The listing builds one solid part. Answer for the finished solid, in the listing's coordinates (mm). Give positions to 0.01 mm unless a question says otherwise; leave off trailing zeros. Order: outer loops, then holes, each group sorted by start corner. A loop starts at its lowest first (then second) coordinate and runs counter-clockwise, first axis right, second up. Notation, with made-up numbers: M 1.25,-11 L 29.25,-11 A17 cw 29.25,5 Z; hole C 68.25,-26.75 d8. An arc over 180 degrees is marked long. Answer as a JSON object with one key per item and string values. Group by question number.
```python
from build123d import *

# Parameters (mm, degrees)
MODEL_R             = 1.6
MODEL_R_2           = 3
MODEL_R_3           = 15
BOSS_EXTRUDE1_DEPTH = 1.5


with BuildPart() as part:
    # Model → Boss-Extrude1 (new, symmetric)
    with BuildSketch(Plane.XY):
        with BuildLine():
            Line((-87, -128), (87, -128))
            ThreePointArc((87, -128), (90.535533906, -126.535533906), (92, -123))
            Line((92, -123), (92, 123))
            ThreePointArc((92, 123), (90.535533906, 126.535533906), (87, 128))
            Line((87, 128), (-87, 128))
            ThreePointArc((-87, 128), (-90.535533906, 126.535533906), (-92, 123))
            Line((-92, 123), (-92, -123))
            ThreePointArc((-92, -123), (-90.535533906, -126.535533906), (-87, -128))
        make_face()
        with Locations((-75, 62)):
            Circle(MODEL_R, mode=Mode.SUBTRACT)
        with Locations((-32, 62)):
            Circle(MODEL_R, mode=Mode.SUBTRACT)
        with Locations((-75, -62)):
            Circle(MODEL_R, mode=Mode.SUBTRACT)
        with Locations((-32, -62)):
            Circle(MODEL_R, mode=Mode.SUBTRACT)
        with Locations((32, 62)):
            Circle(MODEL_R, mode=Mode.SUBTRACT)
        with Locations((75, 62)):
            Circle(MODEL_R, mode=Mode.SUBTRACT)
        with Locations((32, -62)):
            Circle(MODEL_R, mode=Mode.SUBTRACT)
        with Locations((75, -62)):
            Circle(MODEL_R, mode=Mode.SUBTRACT)
        with Locations((-39, 115)):
            Circle(MODEL_R, mode=Mode.SUBTRACT)
        with Locations((-39, 73)):
            Circle(MODEL_R, mode=Mode.SUBTRACT)
        with Locations((39, 115)):
            Circle(MODEL_R, mode=Mode.SUBTRACT)
        with Locations((39, 73)):
            Circle(MODEL_R, mode=Mode.SUBTRACT)
        with Locations((-39, -115)):
            Circle(MODEL_R, mode=Mode.SUBTRACT)
        with Locations((-39, -73)):
            Circle(MODEL_R, mode=Mode.SUBTRACT)
        with Locations((39, -115)):
            Circle(MODEL_R, mode=Mode.SUBTRACT)
        with Locations((39, -73)):
            Circle(MODEL_R, mode=Mode.SUBTRACT)
        Circle(MODEL_R_2, mode=Mode.SUBTRACT)
        with Locations((0, 15)):
            Circle(MODEL_R_2, mode=Mode.SUBTRACT)
        with Locations((0, -15)):
            Circle(MODEL_R_2, mode=Mode.SUBTRACT)
        with Locations((0, 42)):
            Circle(MODEL_R_3, mode=Mode.SUBTRACT)
        with Locations((0, -42)):
            Circle(MODEL_R_3, mode=Mode.SUBTRACT)
        with Locations((-75, 115)):
            Circle(MODEL_R, mode=Mode.SUBTRACT)
        with Locations((75, 115)):
            Circle(MODEL_R, mode=Mode.SUBTRACT)
        with Locations((-75, -115)):
            Circle(MODEL_R, mode=Mode.SUBTRACT)
        with Locations((75, -115)):
            Circle(MODEL_R, mode=Mode.SUBTRACT)
        with Locations((-69, 88.5)):
            Circle(MODEL_R_3, mode=Mode.SUBTRACT)
        with Locations((69, 88.5)):
            Circle(MODEL_R_3, mode=Mode.SUBTRACT)
        with Locations((-69, -88.5)):
            Circle(MODEL_R_3, mode=Mode.SUBTRACT)
        with Locations((69, -88.5)):
            Circle(MODEL_R_3, mode=Mode.SUBTRACT)
        with BuildLine():
            Line((-80.366563146, 62), (-82.4, 62))
            ThreePointArc((-82.4, 62), (-83.53137085, 61.53137085), (-84, 60.4))
            Line((-84, 60.4), (-84, -60.4))
            ThreePointArc((-84, -60.4), (-83.53137085, -61.53137085), (-82.4, -62))
            Line((-82.4, -62), (-80.366563146, -62))
            ThreePointArc((-80.366563146, -62), (-79.410380259, -61.682853961), (-78.83325939, -60.857142857))
            ThreePointArc((-78.83325939, -60.857142857), (-75, -58), (-71.16674061, -60.857142857))
            ThreePointArc((-71.16674061, -60.857142857), (-70.589619741, -61.682853961), (-69.633436854, -62))
            Line((-69.633436854, -62), (-37.366563146, -62))
            ThreePointArc((-37.366563146, -62), (-36.410380259, -61.682853961), (-35.83325939, -60.857142857))
            ThreePointArc((-35.83325939, -60.857142857), (-32, -58), (-28.16674061, -60.857142857))
            ThreePointArc((-28.16674061, -60.857142857), (-27.589619741, -61.682853961), (-26.633436854, -62))
            Line((-26.633436854, -62), (-24.6, -62))
            ThreePointArc((-24.6, -62), (-23.46862915, -61.53137085), (-23, -60.4))
            Line((-23, -60.4), (-23, 60.4))
            ThreePointArc((-23, 60.4), (-23.46862915, 61.53137085), (-24.6, 62))
            Line((-24.6, 62), (-26.633436854, 62))
            ThreePointArc((-26.633436854, 62), (-27.589619741, 61.682853961), (-28.16674061, 60.857142857))
            ThreePointArc((-28.16674061, 60.857142857), (-32, 58), (-35.83325939, 60.857142857))
            ThreePointArc((-35.83325939, 60.857142857), (-36.410380259, 61.682853961), (-37.366563146, 62))
            Line((-37.366563146, 62), (-69.633436854, 62))
            ThreePointArc((-69.633436854, 62), (-70.589619741, 61.682853961), (-71.16674061, 60.857142857))
            ThreePointArc((-71.16674061, 60.857142857), (-75, 58), (-78.83325939, 60.857142857))
            ThreePointArc((-78.83325939, 60.857142857), (-79.410380259, 61.682853961), (-80.366563146, 62))
        make_face(mode=Mode.SUBTRACT)
        with BuildLine():
            Line((26.633436854, 62), (24.6, 62))
            ThreePointArc((24.6, 62), (23.46862915, 61.53137085), (23, 60.4))
            Line((23, 60.4), (23, -60.4))
            ThreePointArc((23, -60.4), (23.46862915, -61.53137085), (24.6, -62))
            Line((24.6, -62), (26.633436854, -62))
            ThreePointArc((26.633436854, -62), (27.589619741, -61.682853961), (28.16674061, -60.857142857))
            ThreePointArc((28.16674061, -60.857142857), (32, -58), (35.83325939, -60.857142857))
            ThreePointArc((35.83325939, -60.857142857), (36.410380259, -61.682853961), (37.366563146, -62))
            Line((37.366563146, -62), (69.633436854, -62))
            ThreePointArc((69.633436854, -62), (70.589619741, -61.682853961), (71.16674061, -60.857142857))
            ThreePointArc((71.16674061, -60.857142857), (75, -58), (78.83325939, -60.857142857))
            ThreePointArc((78.83325939, -60.857142857), (79.410380259, -61.682853961), (80.366563146, -62))
            Line((80.366563146, -62), (82.4, -62))
            ThreePointArc((82.4, -62), (83.53137085, -61.53137085), (84, -60.4))
            Line((84, -60.4), (84, 60.4))
            ThreePointArc((84, 60.4), (83.53137085, 61.53137085), (82.4, 62))
            Line((82.4, 62), (80.366563146, 62))
            ThreePointArc((80.366563146, 62), (79.410380259, 61.682853961), (78.83325939, 60.857142857))
            ThreePointArc((78.83325939, 60.857142857), (75, 58), (71.16674061, 60.857142857))
            ThreePointArc((71.16674061, 60.857142857), (70.589619741, 61.682853961), (69.633436854, 62))
            Line((69.633436854, 62), (37.366563146, 62))
            ThreePointArc((37.366563146, 62), (36.410380259, 61.682853961), (35.83325939, 60.857142857))
            ThreePointArc((35.83325939, 60.857142857), (32, 58), (28.16674061, 60.857142857))
            ThreePointArc((28.16674061, 60.857142857), (27.589619741, 61.682853961), (26.633436854, 62))
        make_face(mode=Mode.SUBTRACT)
        with BuildLine():
            Line((34, 113.6), (34, 74.4))
            ThreePointArc((34, 74.4), (33.121320344, 72.278679656), (31, 71.4))
            Line((31, 71.4), (-31, 71.4))
            ThreePointArc((-31, 71.4), (-33.121320344, 72.278679656), (-34, 74.4))
            Line((-34, 74.4), (-34, 113.6))
            ThreePointArc((-34, 113.6), (-33.121320344, 115.721320344), (-31, 116.6))
            Line((-31, 116.6), (31, 116.6))
            ThreePointArc((31, 116.6), (33.121320344, 115.721320344), (34, 113.6))
        make_face(mode=Mode.SUBTRACT)
        with BuildLine():
            Line((34, -113.6), (34, -74.4))
            ThreePointArc((34, -74.4), (33.121320344, -72.278679656), (31, -71.4))
            Line((31, -71.4), (-31, -71.4))
            ThreePointArc((-31, -71.4), (-33.121320344, -72.278679656), (-34, -74.4))
            Line((-34, -74.4), (-34, -113.6))
            ThreePointArc((-34, -113.6), (-33.121320344, -115.721320344), (-31, -116.6))
            Line((-31, -116.6), (31, -116.6))
            ThreePointArc((31, -116.6), (33.121320344, -115.721320344), (34, -113.6))
        make_face(mode=Mode.SUBTRACT)
    extrude(amount=BOSS_EXTRUDE1_DEPTH, both=True)


solid = part.part
```
Item 1: Consider probe 1 along X at (y, z) = (-115, 0.6); probe 2 along Y at (x, z) = (-39, 0.25); probe 3 along Y at (x, z) = (-20, 0.4). Determine where each line is inside the solid, lowest interval first. Write a range as from..to.
Item 2: Section C-C (y = 100.5) is taken. Determine the outline of the cut face in (x, z).
Item 3: A flat-ended cylindrical pin translates along its axis: P1, Ø2.5, axis at x = 32, y = -62, coming from the +Z side. Find the tip coordinate at first contact, or state that the pin passes through.
Item 4: Section A-A (y = -15) is taken. Determine the outline of the cut face in (x, z), and give its area (3 significant figures).
Item 5: Section B-B (x = 46) is taken. Determine the outline of the cut face in (y, z).
Item 6: Determine the mould class of faces 1 (the cylindrical face through (-1.953, -27.128, -0.021)), 2 (the cylindrical face through (-91, -126, 0)), 3 (the flat face through (6, 1, -1.5)), 4 (the cylindrical face through (65.748, -103.143, -0.021)) for opening direction X: released by +X, released by -X, zero draft, split by the parting line, or undercut.
Item 7: Section D-D (z = -0.95) is taken. Count the separate pieces of the cut face and the enclosed holes in it, and give its area (3 significant figures).
Values found:
{
 "1": {"probe 1": "x = -92..-76.6, -73.4..-40.6, -37.4..-33.65, 33.65..37.4, 40.6..73.4, 76.6..92", "probe 2": "y = -128..-116.6, -113.4..-74.6, -71.4..-62, 62..71.4, 74.6..113.4, 116.6..128", "probe 3": "y = -128..-116.6, -71.4..71.4, 116.6..128"},
 "2": {"outline": "M -92,-1.5 L -78,-1.5 L -78,1.5 L -92,1.5 Z; M -60,-1.5 L -34,-1.5 L -34,1.5 L -60,1.5 Z; M 34,-1.5 L 60,-1.5 L 60,1.5 L 34,1.5 Z; M 78,-1.5 L 92,-1.5 L 92,1.5 L 78,1.5 Z"},
 "3": {"P1": "passes through"},
 "4": {"outline": "M -92,-1.5 L -84,-1.5 L -84,1.5 L -92,1.5 Z; M -23,-1.5 L -3,-1.5 L -3,1.5 L -23,1.5 Z; M 3,-1.5 L 23,-1.5 L 23,1.5 L 3,1.5 Z; M 84,-1.5 L 92,-1.5 L 92,1.5 L 84,1.5 Z", "area": "168 mm^2"},
 "5": {"outline": "M -128,-1.5 L -62,-1.5 L -62,1.5 L -128,1.5 Z; M 62,-1.5 L 128,-1.5 L 128,1.5 L 62,1.5 Z"},
 "6": {"face 1": "undercut", "face 2": "released by -X", "face 3": "zero draft", "face 4": "undercut"},
 "7": {"separate pieces": "1", "enclosed holes": "33", "area": "21,500 mm^2"}
}
